Work out the finished part from the listing and answer in its coordinate system (mm). A direction names the side the tool comes from. Give positions to 0.01 mm unless a question says otherwise; leave off trailing zeros. Order: outer loops, then holes, each group sorted by start corner. A loop starts at its lowest first (then second) coordinate and runs counter-clockwise, first axis right, second up. Notation, with made-up numbers: (74.5, 30) - (113.5, 30) arc R33 ccw to (113.5, 69) - close; hole circle Ø5 at (24.5, 87.5). An arc over 180 degrees is marked (long way). Write each question's results on one line, items separated by ' | '.
Autodesk Inventor part; units mm, degrees
ref_plane "YZ Plane" through (0, 0, 0) normal (1, 0, 0) x (0, 1, 0)
ref_plane "XZ Plane" through (0, 0, 0) normal (0, 1, 0) x (-1, 0, 0)
ref_plane "XY Plane" through (0, 0, 0) normal (0, 0, 1) x (1, 0, 0)
sketch "Sketch1" plane through (0, 0, 0) normal (1, 0, 0) x (0, 1, 0)
  arc A0 (7.3958, -27.6013) -> (7.3958, 27.6013) centre (0, 0) ccw
  line L0 (7.3958, 27.6013) -> (9.6178, 35.894)
  line L1 (0, 0) -> (46.4224, 0) construction
  line L2 (7.3958, -27.6013) -> (9.6178, -35.894)
  line L3 (0, 0) -> (51.2466, 0) construction
  line L4 (30.8102, 20.7753) -> (30.8102, 50.8)
  line L5 (30.8102, 50.8) -> (37.1602, 50.8)
  line L6 (37.1602, 50.8) -> (37.1602, 0)
  line L7 (37.1602, 0) -> (37.1602, -50.8)
  line L8 (37.1602, -50.8) -> (30.8102, -50.8)
  line L9 (30.8102, -50.8) -> (30.8102, -20.7753)
  arc A1 (9.6178, -35.894) -> (30.8102, -20.7753) centre (0, 0) ccw
  arc A2 (30.8102, 20.7753) -> (9.6178, 35.894) centre (0, 0) ccw
extrude "Extrusion1" add sketch "Sketch1" along normal blind 10.16
sketch "Sketch2" plane through (0, 30.8102, 20.7753) normal (0, -1, 0) x (1, 0, 0)
  line L0 (0, 15.1187) -> (10.16, 15.1187)
  line L1 (10.16, -48.3766) -> (10.16, -56.6693)
  line L2 (10.16, 15.1187) -> (10.16, 6.8261)
  circle A0 centre (5.08, 22.5717) radius 1.75
  circle A1 centre (5.08, -64.1223) radius 1.75
  point P0 (0, -20.7753)
  point P1 (10.16, 30.0247)
  point P2 (0, 30.0247)
  point P3 (0, -71.5753)
  dimension "d10" = 3.5
  dimension "d11" = 3.5
extrude "Extrusion2" cut sketch "Sketch2" against normal blind 10.16
sketch "Sketch3" plane through (0, 7.3958, 27.6013) normal (0, -0.9659, 0.2588) x (1, 0, 0)
  circle A0 centre (5.08, 4.2926) radius 2.2
  point P0 (0, -28.575)
  point P1 (0, 8.5852)
  point P2 (10.16, 0)
  dimension "d16" = 4.4
extrude "Extrusion3" cut sketch "Sketch3" against normal blind 4.8
sketch "Sketch4" plane through (0, 9.6178, -35.894) normal (0, -0.9659, -0.2588) x (1, 0, 0)
  circle A0 centre (5.08, 4.2926) radius 2.2
  point P0 (0, 37.1602)
  point P1 (0, 0)
  point P2 (10.16, 8.5852)
extrude "Extrusion4" cut sketch "Sketch4" against normal blind 4.8
fillet "Fillet1" radius 6.35 2 edges at (5.08, 30.8102, -20.7753) (5.08, 30.8102, 20.7753)
chamfer "Chamfer2" distance 1.27 angle 45 10 edges at (10.16, 15.4709, 33.7866) (10.16, 30.8102, 43.3919) (0, 15.4709, 33.7866) (0, 30.8102, 43.3919) (0, 28.575, 0) (10.16, 28.575, 0) (10.16, 15.4709, -33.7866) (10.16, 30.8102, -43.3919) (0, 15.4709, -33.7866) (0, 30.8102, -43.3919)
fillet "Fillet2" radius 3.175 4 edges at (0, 34.6202, 50.8) (10.16, 34.6202, 50.8) (0, 34.6202, -50.8) (10.16, 34.6202, -50.8)
properties part number "bottomCameraMount"
1. Determine the mould class of faces 1 (the face through (5.03, 15.55, -33.75)), 2 (the face through (1.05, 28.79, 0.53)), 3 (the face through (0.91, 34.03, 49.85)), 4 (the face through (5, 37.16, 1)) for opening direction Y: +Y half, -Y half, draft (parallel to the pull), parting line (faces both ways), or undercut.
Answer list:
face 1: undercut | face 2: -Y half | face 3: draft | face 4: +Y half
2. A cutting plane is placed at C-C, the plane z = -39.5. Write down the section's boundary in (x, y).
Answer list:
outline: (0, 32.08) - (1.27, 30.81) - (8.89, 30.81) - (10.16, 32.08) - (10.16, 37.16) - (0, 37.16) - close
3. A tool of negligible diameter and unlimited length cuts with its end or side. For faces 5 (the face through (5, 15, 34)), 6 (the face through (4, 30.81, 45)), 7 (the face through (5.05, 13.15, 30.53)), from which of +Z, -Z, +X, -X, +Y, -Y can it reach the whole face along a straight path? Write none if from no direction.
Answer list:
face 5: +Z, +X, -X | face 6: +Z, +X, -X, -Y | face 7: none
4. A cutting plane is placed at A-A, the plane x = 5.08. Write down the section's boundary in (y, z), then the cut area to 3 significant figures.
Answer list:
outline: (7.4, -27.6) - (7.94, -29.62) - (12.58, -28.38) - (13.71, -32.63) - (9.08, -33.87) - (9.62, -35.89) arc R37.16 ccw to (20.89, -30.73) arc R6.35 cw to (30.81, -35.98) - (30.81, -41.6) - (37.16, -41.6) - (37.16, 41.6) - (30.81, 41.6) - (30.81, 35.98) arc R6.35 cw to (20.89, 30.73) arc R37.16 ccw to (9.62, 35.89) - (9.08, 33.87) - (13.71, 32.63) - (12.58, 28.38) - (7.94, 29.62) - (7.4, 27.6) arc R28.57 cw to start; (30.81, -50.8) - (37.16, -50.8) - (37.16, -45.1) - (30.81, -45.1) - close; (30.81, 45.1) - (37.16, 45.1) - (37.16, 50.8) - (30.81, 50.8) - close | area: 1,200 mm^2
5. Straight lines are drawn through the part: line 1 (Z direction, x = 5.08, y = 33.5); line 2 (Y direction, x = 8.25, z = 39); line 3 (Y direction, x = 7.5, z = -33.5). For each, find the intervals that lie inside material, in ascending order. Write a range as [from, to].
Answer list:
line 1: [-50.8, -45.1], [-41.6, 41.6], [45.1, 50.8] | line 2: [30.81, 37.16] | line 3: [8.98, 16.08], [30.3, 37.16]
6. A cutting plane is placed at B-B, the plane y = 33.25. Write down the section's boundary in (x, z) (3 decimals).
Answer list:
outline: (0, -47.625) arc R3.175 ccw to (3.175, -50.8) - (6.985, -50.8) arc R3.175 ccw to (10.16, -47.625) - (10.16, 47.625) arc R3.175 ccw to (6.985, 50.8) - (3.175, 50.8) arc R3.175 ccw to (0, 47.625) - close; hole circle Ø3.5 at (5.08, -43.347); hole circle Ø3.5 at (5.08, 43.347)
7. Given P1, Ø6, axis at x = 6.5, z = -12, coming from the -Y side; P2, Ø1.5, axis at x = 9, z = 8, coming from the -Y side; P3, Ø6, axis at x = 5.5, z = 41.5, coming from the -Y side, each flat-ended and moving along its own axis, determine where each tip first touches the part or whether it passes through.
Answer list:
P1: y = 24.32 | P2: y = 27.2 | P3: y = 30.81
